The listing builds one solid part. Answer for the finished solid, in the listing's coordinates (mm). A direction names the side the tool comes from. Coordinates: 2 decimals unless noted, no trailing zeros. Order: outer loops, then holes, each group sorted by start corner. A loop starts at its lowest first (then second) coordinate and runs counter-clockwise, first axis right, second up.
from build123d import *

# Parameters (mm, degrees)
SKETCH_1_W      = 30
SKETCH_1_H      = 18
EXTRUDE_1_DEPTH = 3
SKETCH_2_W      = 30
SKETCH_2_H      = 3
EXTRUDE_2_DEPTH = 7
FILLET_1_R      = 2
SKETCH_5_W      = 30
SKETCH_5_H      = 2.5
EXTRUDE_3_DEPTH = 12.5


with BuildPart() as part:
    # 스케치1 → 보스-돌출1 (new body)
    with BuildSketch(Plane(origin=(0, 0, 0), x_dir=(1, 0, 0), z_dir=(0, 1, 0))):
        Rectangle(SKETCH_1_W, SKETCH_1_H)
    extrude(amount=EXTRUDE_1_DEPTH)

    # 스케치2 → 보스-돌출2 (add)
    with BuildSketch(Plane.XZ):
        with Locations((0, 7.5)):
            Rectangle(SKETCH_2_W, SKETCH_2_H)
    extrude(amount=EXTRUDE_2_DEPTH)

    # 필렛1
    fillet_1_edges = [part.edges().sort_by_distance(p)[0] for p in [
        (0, 3, 9),
    ]]
    fillet(fillet_1_edges, radius=FILLET_1_R)

    # 스케치5 → 보스-돌출3 (add)
    with BuildSketch(Plane(origin=(0, 3, 0), x_dir=(1, 0, 0), z_dir=(0, 1, 0))):
        with Locations((0, 7.75)):
            Rectangle(SKETCH_5_W, SKETCH_5_H)
    extrude(amount=EXTRUDE_3_DEPTH)


solid = part.part
1) Section A-A (x = 7) is taken. Give the vertices of the cut face in (y, z).
2) Section C-C (z = -3.25) is taken. Give the vertices of the cut face in (x, y).
3) Consider L1, parallel to Y at x = 5.25, z = -5.25; L2, parallel to Z at x = -2.5, y = 4.75; L3, parallel to Y at x = 5.5, z = 6.75. Determine where each line is inside the solid, lowest interval first.
4) Section B-B (y = 11) is taken. Give the vertices of the cut face in (x, z), then the cut area to 3 significant figures.
5) Each of these flat-tipped pins is pushed along its axis until it touches: P1, Ø8, axis at x = -2.5, z = 0, coming from the -Y side; P2, Ø5.5, axis at x = 1, y = -3, coming from the -Z side; P3, Ø6, axis at x = 7, y = 7.5, coming from the +Z side; P4, Ø5, axis at y = 7.5, z = -3, coming from the +X side. Where does it stop, or does it pass through?
6) A tool of negligible diameter and unlimited length cuts with its end or side. For faces 1 (the face through (0, 8, -9)), 2 (the face through (0, -3, 6)), 3 (the face through (0, 9, -6.5)), from which of +Z, -Z, +X, -X, +Y, -Y can it reach the whole face along a straight path? Write none if from no direction.
Filled sheet:
1. outline: (-7, 6) - (0, 6) - (0, -9) - (15.5, -9) - (15.5, -6.5) - (3, -6.5) - (3, 7) arc R2 ccw to (1, 9) - (-7, 9) - close
2. outline: (-15, 0) - (15, 0) - (15, 3) - (-15, 3) - close
3. L1: y = 0 to 3
3. L2: z = -9 to -6.5
3. L3: y = -7 to 3
4. outline: (-15, -9) - (15, -9) - (15, -6.5) - (-15, -6.5) - close
4. area: 75.0 mm2
5. P1: stops at y = 0
5. P2: stops at z = 6
5. P3: stops at z = -6.5
5. P4: passes through
6. face 1: -Z, +X, -X, +Y, -Y
6. face 2: -Z, +X, -X, -Y
6. face 3: +Z, +X, -X, +Y
